The model under review builds one solid part; all positions refer to its coordinate system, in mm. A direction names the side the tool comes from. Round coordinates to 2 decimals unless told otherwise and drop trailing zeros. Write each loop counter-clockwise with the first axis right and the second up, starting at its lowest first coordinate (ties: lowest second). Pieces come first, ordered by that corner, then holes. Notation, with made-up numbers: (27, 67.5) - (58, 67.5) arc R28 cw to (58, 102.5) - close; hole circle Ø11 at (-37, -6). An arc over 180 degrees is marked (long way). Use one line per item in the form item = value.
from build123d import *

# Parameters (mm, degrees)
BOSS_EXTRU_1_DEPTH = 5
CUT_EXTRUDE1_DEPTH = 10


with BuildPart() as part:
    # Esquisse1 → Boss.-Extru.1 (new body)
    with BuildSketch(Plane.XY):
        Polygon((3.468077367, 2.92543021), (8.468077367, 2.92543021), (8.468077367, -43.07456979), (3.468077367, -43.07456979), (3.468077367, -38.07456979), (-1.531922633, -38.07456979), (-1.531922633, -43.07456979), (-6.531922633, -43.07456979), (-6.531922633, 2.92543021), (-1.531922633, 2.92543021), (-1.531922633, -2.07456979), (3.468077367, -2.07456979), align=None)
    extrude(amount=BOSS_EXTRU_1_DEPTH)

    # Esquisse2 → Cut-Extrude1 (cut)
    with BuildSketch(Plane(origin=(0, 0, 0), x_dir=(-1, 0, 0), z_dir=(0, 0, -1))):
        Polygon((-3.468077367, -21.517945463), (-0.968077367, -22.961321136), (1.531922633, -21.517945463), (1.531922633, -18.631194117), (-0.968077367, -17.187818444), (-3.468077367, -18.631194117), align=None)
    extrude(amount=-CUT_EXTRUDE1_DEPTH, mode=Mode.SUBTRACT)


solid = part.part
(1) The part is to be moulded in two halves that separate along Y. For faces 4 (the flat face through (-4, 2.925, 2)), 5 (the flat face through (-0.3, -17.92, 2.46)), 6 (the flat face through (-4, -43.075, 2)), say which applies: +Y half, -Y half, draft (parallel to the pull), parting line (faces both ways), or undercut.
Geometry results:
face_4 = +Y half
face_5 = undercut
face_6 = -Y half
(2) Add section B-B on x = -0.75. Write out the cut boundary in (y, z), then the cut area to 3 significant figures.
Geometry results:
outline = (-38.07, 0) - (-21.97, 0) - (-21.97, 5) - (-38.07, 5) - close; (-18.18, 0) - (-2.07, 0) - (-2.07, 5) - (-18.18, 5) - close
area = 161 mm2
(3) Machinability: for faces 1 (the flat face through (3.468, -20, 2)), 2 (the flat face through (-1.532, 0, 2)), 3 (the flat face through (3.468, -41, 2)), which of the approach directions +Z, -Z, +X, -X, +Y, -Y give a long, thin tool a straight path to every point of the face, cutting with its end or side? Answer none if there is none.
Geometry results:
face_1 = +Z, -Z
face_2 = +Z, -Z, +Y
face_3 = +Z, -Z, -Y
(4) Add section A-A on z = 2.9. Write out the cut boundary in (x, y), then the cut area to 3 significant figures.
Geometry results:
outline = (-6.53, -43.07) - (-1.53, -43.07) - (-1.53, -38.07) - (3.47, -38.07) - (3.47, -43.07) - (8.47, -43.07) - (8.47, 2.93) - (3.47, 2.93) - (3.47, -2.07) - (-1.53, -2.07) - (-1.53, 2.93) - (-6.53, 2.93) - close; hole (-1.53, -21.52) - (0.97, -22.96) - (3.47, -21.52) - (3.47, -18.63) - (0.97, -17.19) - (-1.53, -18.63) - close
area = 618 mm2
(5) Insertion check: P1, Ø1.5, axis at x = 0.5, z = 2, coming from the -Y side; P2, Ø2.5, axis at x = 0.5, z = 1.5, coming from the +Y side. Each pin has a flat end and moves straight along its axis. Give the tip position at first contact, or say it passes through.
Geometry results:
P1 = -38.07
P2 = -2.07
(6) To check wall thickness, follow L1, parallel to X at y = -19, z = 3.4; L2, parallel to Y at x = -0.75, z = 4.35; L3, parallel to Y at x = 3.25, z = 1.35. State the ranges of each line that lie inside material, in increasing order.
Geometry results:
L1 = -6.53 to -1.53, 3.47 to 8.47
L2 = -38.07 to -21.97, -18.18 to -2.07
L3 = -38.07 to -21.64, -18.51 to -2.07
